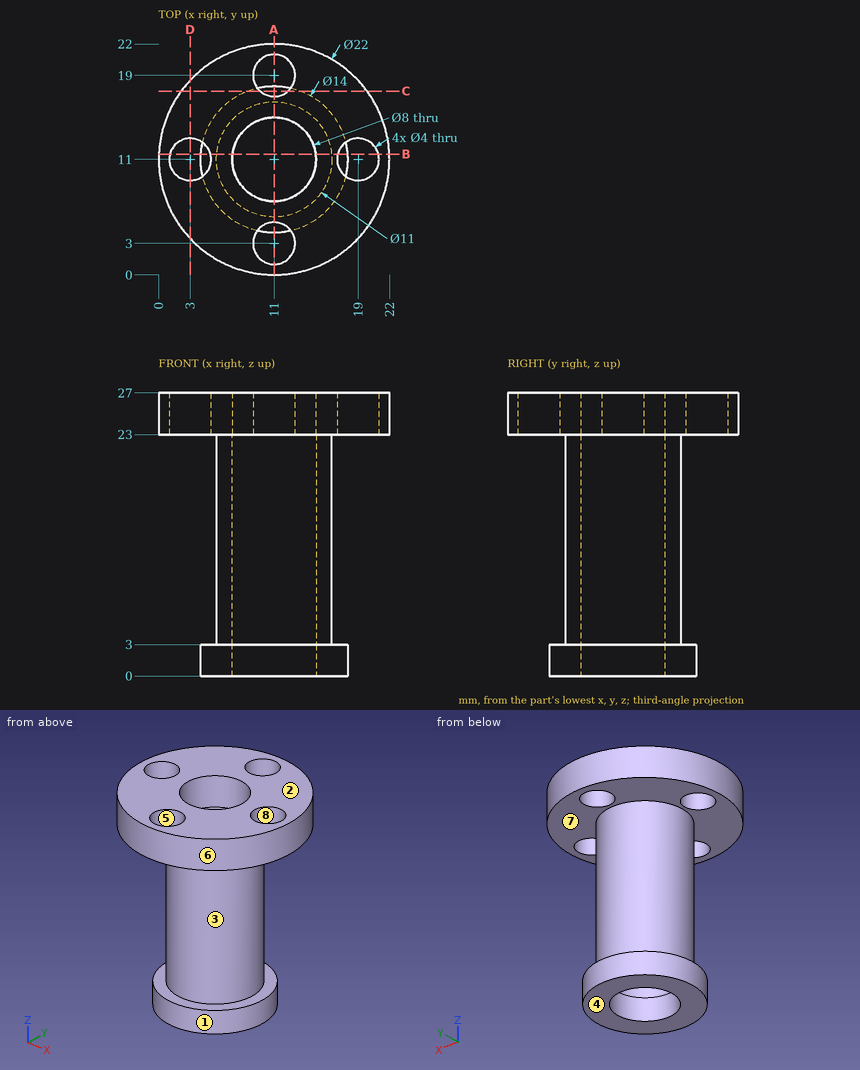
Source: three-view drawing plus pictorial views. Frame: mm from the lowest corner of the part. A direction names the side the tool comes from. Coordinates: 2 decimals unless noted, no trailing zeros. Loops run counter-clockwise (first coordinate to the right, second up) from the corner with the lowest first, then second, coordinate; pieces in that order, holes last. Notation, with made-up numbers: (-18.5, 8) -> (-7.5, 8) arc R31 cw to (-7.5, 44) -> close; hole circle Ø9 at (7, 83.5). An arc over 180 degrees is marked (long way). Answer in a Markdown table with one row per item. Add a question column.
Q1. Reachability of the marked faces 1, 2, 3, 4 and 5 from +Z, -Z, +X, -X, +Y, -Y: full face, straight path, thin tool, end or side. Return the list, or none.
Q2. Contact query for flat-ended pins moving along their axis: pin 1 Ø3 at (x, y) = (19, 11) entering from +Z; pin 2 Ø3 at (y, z) = (14.5, 14) entering from -X; pin 3 Ø8 at (y, z) = (14.5, 11) entering from -X; pin 4 Ø7 at (x, y) = (11, 11) entering from -Z. Output: stop coordinate, or through.
Q3. Section A-A on x = 11. Return the cut outline in (y, z).
Q4. Section C-C on y = 17.5. Return the cut outline in (x, z).
Q5. Section D-D on x = 3. Return the cut outline in (y, z).
Q6. Ray query, line 1 along Y through (x, z) = (11, 24.55); line 2 along Z through (x, y) = (15.5, 15); line 3 along Z through (x, y) = (6.5, 2). Return the intervals inside material, ascending.
Q7. Pull-direction query (Y, two-part tool) for the marked faces 6, 7 and 8; classes: pulls with the +Y half, pulls with the -Y half, needs draft (parallel to the pull), parting line crosses it, or undercut.
Q8. Section B-B on y = 11.5. Return the cut outline in (x, z).
Computed values:
| question | item | result |
|---|---|---|
| 1 | face 1 | -Z |
| 1 | face 2 | +Z, +X, -X, +Y, -Y |
| 1 | face 3 | none |
| 1 | face 4 | -Z, +X, -X, +Y, -Y |
| 1 | face 5 | +Z |
| 2 | pin 1 | stops at z = 3 |
| 2 | pin 2 | stops at x = 5.88 |
| 2 | pin 3 | stops at x = 5.5 |
| 2 | pin 4 | passes through |
| 3 | outline | (0, 23) -> (1, 23) -> (1, 27) -> (0, 27) -> close; (4, 0) -> (7, 0) -> (7, 27) -> (5, 27) -> (5, 23) -> (5.5, 23) -> (5.5, 3) -> (4, 3) -> close; (15, 0) -> (18, 0) -> (18, 3) -> (16.5, 3) -> (16.5, 23) -> (17, 23) -> (17, 27) -> (15, 27) -> close; (21, 23) -> (22, 23) -> (22, 27) -> (21, 27) -> close |
| 4 | outline | (2.13, 23) -> (9.68, 23) -> (9.68, 27) -> (2.13, 27) -> close; (8.4, 0) -> (13.6, 0) -> (13.6, 3) -> (8.4, 3) -> close; (12.32, 23) -> (19.87, 23) -> (19.87, 27) -> (12.32, 27) -> close |
| 5 | outline | (3.45, 23) -> (9, 23) -> (9, 27) -> (3.45, 27) -> close; (13, 23) -> (18.55, 23) -> (18.55, 27) -> (13, 27) -> close |
| 6 | line 1 | y = 0 to 1, 5 to 7, 15 to 17, 21 to 22 |
| 6 | line 2 | z = 0 to 3, 23 to 27 |
| 6 | line 3 | z = 23 to 27 |
| 7 | face 6 | parting line crosses it |
| 7 | face 7 | needs draft |
| 7 | face 8 | undercut |
| 8 | outline | (0.01, 23) -> (1.06, 23) -> (1.06, 27) -> (0.01, 27) -> close; (4.02, 0) -> (7.03, 0) -> (7.03, 27) -> (4.94, 27) -> (4.94, 23) -> (5.52, 23) -> (5.52, 3) -> (4.02, 3) -> close; (14.97, 0) -> (17.98, 0) -> (17.98, 3) -> (16.48, 3) -> (16.48, 23) -> (17.06, 23) -> (17.06, 27) -> (14.97, 27) -> close; (20.94, 23) -> (21.99, 23) -> (21.99, 27) -> (20.94, 27) -> close |
